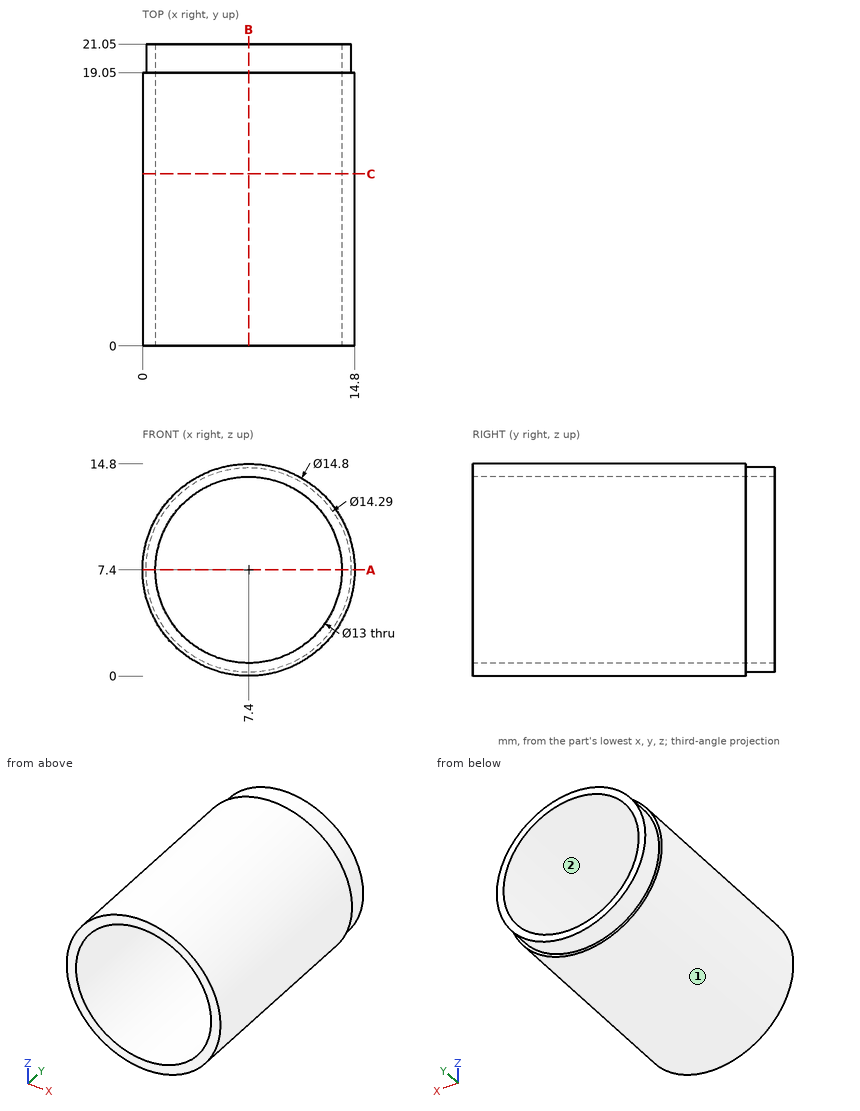
Geometry: see drawing. Coordinates: mm, zero at the bounding-box minimum. Round coordinates to 2 decimals unless told otherwise and drop trailing zeros. Loops run counter-clockwise (first coordinate to the right, second up) from the corner with the lowest first, then second, coordinate; pieces in that order, holes last. Notation, with made-up numbers: (51.5, -33.5) -> (73.5, -33.5) arc R23 cw to (73.5, 5.5) -> close; hole circle Ø7 at (-22.75, -3). An arc over 180 degrees is marked (long way). Use one line per item in the form item = value. Start each with the question number.
Item 1: Section query B-B on x = 7.4. Return the cut outline in (y, z) (3 decimals), then the cut area to 3 significant figures.
Item 2: Section query C-C on y = 12. Return the cut outline in (x, z), then the cut area to 3 significant figures.
Item 3: Material intervals for L1, parallel to Z at x = 7.4, y = 7.75; L2, parallel to X at y = 19.75, z = 7.5, sorted ascending. Write a range as from..to.
Item 4: Contact query for flat-ended pins moving along their axis: pin 1 Ø4 at (y, z) = (4, 12.5) entering from +X; pin 2 Ø6 at (y, z) = (8, 3) entering from +X. Output: stop coordinate, or through.
Item 5: Mould query, pull axis X, two halves, no side actions, for the marked faces 1 and 2. Classes: pulls with the +X half, pulls with the -X half, needs draft (parallel to the pull), parting line crosses it, or undercut.
Item 6: Section query A-A on z = 7.4. Return the cut outline in (x, y) (3 decimals).
Ans:
q1.outline = (0, 0) -> (19.05, 0) -> (19.05, 0.255) -> (21.05, 0.255) -> (21.05, 0.9) -> (0, 0.9) -> close; (0, 13.9) -> (21.05, 13.9) -> (21.05, 14.545) -> (19.05, 14.545) -> (19.05, 14.8) -> (0, 14.8) -> close
q1.area = 36.9 mm^2
q2.outline = circle Ø14.8 at (7.4, 7.4); hole circle Ø13 at (7.4, 7.4)
q2.area = 39.3 mm^2
q3.L1 = 0..0.9, 13.9..14.8
q3.L2 = 0.26..0.9, 13.9..14.54
q4.pin_1 = 14.12
q4.pin_2 = 14.67
q5.face_1 = parting line crosses it
q5.face_2 = undercut
q6.outline = (0, 0) -> (0.9, 0) -> (0.9, 21.05) -> (0.255, 21.05) -> (0.255, 19.05) -> (0, 19.05) -> close; (13.9, 0) -> (14.8, 0) -> (14.8, 19.05) -> (14.545, 19.05) -> (14.545, 21.05) -> (13.9, 21.05) -> close
